Here's how the part is built. I have some questions about the finished solid (model axes, mm). A direction names the side the tool comes from. Coordinates: 2 decimals unless noted, no trailing zeros. Write each loop counter-clockwise with the first axis right and the second up, starting at its lowest first coordinate (ties: lowest second). Pieces come first, ordered by that corner, then holes. Notation, with made-up numbers: (17.5, 63.25) -> (68.5, 63.25) arc R15 cw to (68.5, 75.25) -> close; hole circle Ø4 at (3, -15). An arc over 180 degrees is marked (long way). Use a Markdown table: item, result. Add a question column.
```python
from build123d import *

# Parameters (mm, degrees)
FILLET1_R           = 0.79375
BOSS_EXTRUDE1_DEPTH = 20
CUT_EXTRUDE1_DEPTH  = 7.35


with BuildPart() as part:
    # Sketch1 → Revolve1 (revolve)
    with BuildSketch(Plane(origin=(0, 0, 0), x_dir=(0, 0, -1), z_dir=(1, 0, 0))):
        Polygon((22.225, 9.525), (22.225, 3.175), (25.4, 3.175), (25.4, -3.175), (6.35, -3.175), (6.35, 3.175), (19.05, 3.175), (19.05, 9.525), align=None)
    revolve(axis=Axis((0, -32.325211936, 0), (0, 1, 0)))

    # Fillet1
    fillet1_edges = [part.edges().sort_by_distance(p)[0] for p in [
        (0, 9.525, 22.225),
        (0, 3.175, 6.35),
        (0, -3.175, 6.35),
    ]]
    fillet(fillet1_edges, radius=FILLET1_R)

    # Sketch2 → Boss-Extrude1 (add, symmetric)
    with BuildSketch(Plane(origin=(0, 0, 0), x_dir=(0, 0, -1), z_dir=(1, 0, 0))):
        Polygon((25.4, 3.175), (12.7, 3.175), (12.7, -3.175), (19.05, -3.175), (19.05, -23.174999878), (25.4, -23.174999878), (25.4, -3.175), align=None)
    extrude(amount=BOSS_EXTRUDE1_DEPTH, both=True)

    # Sketch3 → Cut-Extrude1 (cut, through all)
    with BuildSketch(Plane.XY.offset(-19.05)):
        with BuildLine():
            ThreePointArc((-10, -11.075), (-12.1, -13.175), (-10, -15.275))
            ThreePointArc((-10, -15.275), (-8.51507576, -14.65992424), (-7.9, -13.175))
            ThreePointArc((-7.9, -13.175), (-8.51507576, -11.69007576), (-10, -11.075))
        make_face()
        with BuildLine():
            ThreePointArc((10, -11.075), (7.9, -13.175), (10, -15.275))
            ThreePointArc((10, -15.275), (11.48492424, -14.65992424), (12.1, -13.175))
            ThreePointArc((12.1, -13.175), (11.48492424, -11.69007576), (10, -11.075))
        make_face()
    extrude(amount=-CUT_EXTRUDE1_DEPTH, mode=Mode.SUBTRACT)


solid = part.part
```
Q1. Please list where these lines run through material, in increasing order: line 1 (X direction, y = -1, z = 0); line 2 (Z direction, x = 0, y = 5) (3 decimals).
Q2. Which directions (+Z, -Z, +X, -X, +Y, -Y) give clear straight access to the entire face, cutting with the end or side of a thin tool? Please do faces 1 (the flat face through (20, -10, -22)), 2 (the cylindrical face through (-6.676, 5.914, -21.199)), 3 (the flat face through (0, -13, -19.05)), 4 (the flat face through (-20, -10, -22)).
Q3. Suppose I cut it at C-C, the plane y = -1.5. Write out the boundary of the cut face in (x, z).
Q4. Suppose I cut it at D-D, the plane y = -12.5. Write out the boundary of the cut face in (x, z).
Q5. Thinking about a two-plate mould opening in X: for faces 5 (the flat face through (0, -3.175, 8)), 6 (the cylindrical face through (6.2, 0.03, 1.38)), 7 (the flat face through (8, 3.175, 0)), 8 (the cylindrical face through (-0.795, -0.044, 25.388)), which applies, released by +X, released by -X, zero draft, split by the parting line, or undercut?
Q6. Will these pins go through, and if not, where does the flat tip stop? pin 1 (8 mm diameter, centred on x = -11, y = -8.5, fed in from +Z); pin 2 (10.5 mm diameter, centred on y = -3.5, z = -21, fed in from +X); pin 3 (22 mm diameter, centred on x = -7, z = -4, fed in from -Y) (3 decimals); pin 4 (1.5 mm diameter, centred on x = 3.5, z = 2.5, fed in from -Y).
Answer key:
| question | item | result |
|---|---|---|
| 1 | line 1 | x = -25.4 to -6.35, 6.35 to 25.4 |
| 1 | line 2 | z = -22.225 to -19.05, 19.05 to 22.225 |
| 2 | face 1 | -Z, +X, +Y, -Y |
| 2 | face 2 | +Y |
| 2 | face 3 | +Z, +X, -X, -Y |
| 2 | face 4 | -Z, -X, +Y, -Y |
| 3 | outline | (-20, -25.4) -> (20, -25.4) -> (20, -15.66) arc R25.4 ccw (long way) to (-20, -15.66) -> close; hole circle Ø12.7 at (0, 0) |
| 4 | outline | (-20, -25.4) -> (-11.99, -25.4) -> (-11.99, -19.05) -> (-20, -19.05) -> close; (-8.01, -25.4) -> (8.01, -25.4) -> (8.01, -19.05) -> (-8.01, -19.05) -> close; (11.99, -25.4) -> (20, -25.4) -> (20, -19.05) -> (11.99, -19.05) -> close |
| 5 | face 5 | zero draft |
| 5 | face 6 | undercut |
| 5 | face 7 | undercut |
| 5 | face 8 | split by the parting line |
| 6 | pin 1 | stops at z = -19.05 |
| 6 | pin 2 | stops at x = 20 |
| 6 | pin 3 | stops at y = -3.175 |
| 6 | pin 4 | passes through |
